Check sheet for the modelled part. Datum: model origin and axes. Units: mm. A direction names the side the tool comes from. Coordinates: 2 decimals unless noted, no trailing zeros. Write each loop counter-clockwise with the first axis right and the second up, starting at its lowest first coordinate (ties: lowest second). Pieces come first, ordered by that corner, then holes. Notation, with made-up numbers: M 2,-23.5 L 15,-23.5 A16 cw 15,-12.5 Z; hole C -14.5,-23 d6. An arc over 180 degrees is marked long. Answer as CSV lines item,"result". Start each with the question number.
1) Go/stop test with flat-tipped pins: pin 1 Ø5.5 at (x, z) = (0, 0) entering from -Y; pin 2 Ø3 at (x, y) = (-2, 13.5) entering from +Z; pin 3 Ø3 at (x, y) = (-3, 8.5) entering from +Z; pin 4 Ø5 at (x, y) = (-2.5, 7.5) entering from -Z. Record where each tip stops, or that it passes through.
2) Draft check along Z on faces 1 (the cylindrical face through (-2.579, 6.162, 1.978)), 2 (the flat face through (1.4, 0, 1.4)), 3 (the flat face through (1.496, 17.993, -0.816)), 4 (the flat face through (0, 2.5, 0)). Enter one of: +Z half, -Z half, draft (parallel to the pull), parting line (faces both ways), or undercut.
3) Section check B-B (y = 11). Record the cut outline in (x, z).
4) Material ranges on L1, parallel to Z at x = 0, y = 0.9; L2, parallel to Y at x = 1, z = -0.75; L3, parallel to Y at x = 0.75, z = -3.5, recorded low to high. Write a range as [from, to].
5) Section check A-A (z = 0). Record the cut outline in (x, y).
6) Access from +Z, -Z, +X, -X, +Y, -Y to the whole of each face (thin tool, end or side, straight path). Record for faces 5 (the flat face through (0, 18, 1.703)), 6 (the cylindrical face through (1.617, 1.232, -0.67)), 7 (the flat face through (-1.454, 17.993, -0.887)).
7) Section check C-C (y = 15). Record the cut outline in (x, z).
from build123d import *

# Parameters (mm, degrees)
SKETCH1_R           = 3.25
BOSS_EXTRUDE1_DEPTH = 12.5
SKETCH2_R           = 1.75
CUT_EXTRUDE1_DEPTH  = 2.5
SKETCH6_R           = 4.8
BOSS_EXTRUDE2_DEPTH = 5
BOSS_EXTRUDE5_DEPTH = 1
FILLET1_R           = 0.75


with BuildPart() as part:
    # Sketch1 → Boss-Extrude1 (new body)
    with BuildSketch(Plane(origin=(0, 0, 0), x_dir=(1, 0, 0), z_dir=(0, 1, 0))):
        Circle(SKETCH1_R)
    extrude(amount=BOSS_EXTRUDE1_DEPTH)

    # Sketch2 → Cut-Extrude1 (cut)
    with BuildSketch(Plane.XZ):
        Circle(SKETCH2_R)
    extrude(amount=-CUT_EXTRUDE1_DEPTH, mode=Mode.SUBTRACT)

    # Sketch6 → Boss-Extrude2 (add)
    with BuildSketch(Plane(origin=(0, 12.5, 0), x_dir=(1, 0, 0), z_dir=(0, 1, 0))):
        Circle(SKETCH6_R)
    extrude(amount=BOSS_EXTRUDE2_DEPTH)

    # Sketch7 → Boss-Extrude5 (add)
    with BuildSketch(Plane(origin=(0, 17.5, 0), x_dir=(1, 0, 0), z_dir=(0, 1, 0))):
        Polygon((2.95, -1.703183294), (0, 3.406366588), (-2.95, -1.703183294), align=None)
    extrude(amount=BOSS_EXTRUDE5_DEPTH)

    # Fillet1
    fillet1_edges = [part.edges().sort_by_distance(p)[0] for p in [
        (-4.8, 17.5, 0),
    ]]
    fillet(fillet1_edges, radius=FILLET1_R)


solid = part.part
Results found:
1,pin 1,"stops at y = 0"
1,pin 2,"stops at z = 4.77"
1,pin 3,"stops at z = 2.88"
1,pin 4,"stops at z = -3.25"
2,face 1,"parting line"
2,face 2,"draft"
2,face 3,"-Z half"
2,face 4,"undercut"
3,outline,"C 0,0 d6.5"
4,L1,"z = [-3.25, -1.75], [1.75, 3.25]"
4,L2,"y = [2.5, 18.5]"
4,L3,"y = [12.5, 17.5]"
5,outline,"M -4.8,12.5 L -3.25,12.5 L -3.25,0 L -1.75,0 L -1.75,2.5 L 1.75,2.5 L 1.75,0 L 3.25,0 L 3.25,12.5 L 4.8,12.5 L 4.8,16.75 A0.75 ccw 4.05,17.5 L 1.97,17.5 L 1.97,18.5 L -1.97,18.5 L -1.97,17.5 L -4.05,17.5 A0.75 ccw -4.8,16.75 Z"
6,face 5,"+Z, +X, -X, +Y"
6,face 6,"-Y"
6,face 7,"-Z, -X, +Y"
7,outline,"C 0,0 d9.6"
